from build123d import *

# Parameters (mm, degrees)
SKETCH1_W           = 139.7
SKETCH1_H           = 292.1
BOSS_EXTRUDE1_DEPTH = 6.35
FILLET1_R           = 12.7
SKETCH2_W           = 7.62
SKETCH2_H           = 29.0068
CUT_EXTRUDE1_DEPTH  = 6.35


with BuildPart() as part:
    # Sketch1 → Boss-Extrude1 (new body)
    with BuildSketch(Plane.XY):
        Rectangle(SKETCH1_W, SKETCH1_H)
    extrude(amount=BOSS_EXTRUDE1_DEPTH)

    # Fillet1
    fillet1_edges = [part.edges().sort_by_distance(p)[0] for p in [
        (69.85, -146.05, 3.175),
        (-69.85, -146.05, 3.175),
        (-69.85, 146.05, 3.175),
        (69.85, 146.05, 3.175),
    ]]
    fillet(fillet1_edges, radius=FILLET1_R)

    # Sketch2 → Cut-Extrude1 (cut)
    with BuildSketch(Plane.XY.offset(6.35)):
        with Locations((52.50815, 119.8626)):
            Rectangle(SKETCH2_W, SKETCH2_H)
        with BuildLine():
            Line((48.69815, 134.366), (56.31815, 134.366))
            ThreePointArc((56.31815, 134.366), (52.50815, 138.176), (48.69815, 134.366))
        make_face()
        with BuildLine():
            Line((48.69815, 105.3592), (56.31815, 105.3592))
            ThreePointArc((56.31815, 105.3592), (52.50815, 101.5492), (48.69815, 105.3592))
        make_face()
        with BuildLine():
            Line((48.69815, 65.6844), (48.69815, 94.6912))
            ThreePointArc((48.69815, 94.6912), (52.50815, 98.5012), (56.31815, 94.6912))
            Line((56.31815, 94.6912), (56.31815, 65.6844))
            ThreePointArc((56.31815, 65.6844), (52.50815, 61.8744), (48.69815, 65.6844))
        make_face()
        with BuildLine():
            Line((-56.31815, 65.6844), (-56.31815, 94.6912))
            ThreePointArc((-56.31815, 94.6912), (-52.50815, 98.5012), (-48.69815, 94.6912))
            Line((-48.69815, 94.6912), (-48.69815, 65.6844))
            ThreePointArc((-48.69815, 65.6844), (-52.50815, 61.8744), (-56.31815, 65.6844))
        make_face()
        with BuildLine():
            Line((-56.31815, 105.3592), (-56.31815, 134.366))
            ThreePointArc((-56.31815, 134.366), (-52.50815, 138.176), (-48.69815, 134.366))
            Line((-48.69815, 134.366), (-48.69815, 105.3592))
            ThreePointArc((-48.69815, 105.3592), (-52.50815, 101.5492), (-56.31815, 105.3592))
        make_face()
        with BuildLine():
            Line((48.69815, 26.0096), (48.69815, 55.0164))
            ThreePointArc((48.69815, 55.0164), (52.50815, 58.8264), (56.31815, 55.0164))
            Line((56.31815, 55.0164), (56.31815, 26.0096))
            ThreePointArc((56.31815, 26.0096), (52.50815, 22.1996), (48.69815, 26.0096))
        make_face()
        with BuildLine():
            Line((-56.31815, 26.0096), (-56.31815, 55.0164))
            ThreePointArc((-56.31815, 55.0164), (-52.50815, 58.8264), (-48.69815, 55.0164))
            Line((-48.69815, 55.0164), (-48.69815, 26.0096))
            ThreePointArc((-48.69815, 26.0096), (-52.50815, 22.1996), (-56.31815, 26.0096))
        make_face()
        with BuildLine():
            Line((48.69815, -13.6652), (48.69815, 15.3416))
            ThreePointArc((48.69815, 15.3416), (52.50815, 19.1516), (56.31815, 15.3416))
            Line((56.31815, 15.3416), (56.31815, -13.6652))
            ThreePointArc((56.31815, -13.6652), (52.50815, -17.4752), (48.69815, -13.6652))
        make_face()
        with BuildLine():
            Line((-56.31815, -13.6652), (-56.31815, 15.3416))
            ThreePointArc((-56.31815, 15.3416), (-52.50815, 19.1516), (-48.69815, 15.3416))
            Line((-48.69815, 15.3416), (-48.69815, -13.6652))
            ThreePointArc((-48.69815, -13.6652), (-52.50815, -17.4752), (-56.31815, -13.6652))
        make_face()
        with BuildLine():
            Line((-56.31815, -53.34), (-56.31815, -24.3332))
            ThreePointArc((-56.31815, -24.3332), (-52.50815, -20.5232), (-48.69815, -24.3332))
            Line((-48.69815, -24.3332), (-48.69815, -53.34))
            ThreePointArc((-48.69815, -53.34), (-52.50815, -57.15), (-56.31815, -53.34))
        make_face()
        with BuildLine():
            Line((48.69815, -53.34), (48.69815, -24.3332))
            ThreePointArc((48.69815, -24.3332), (52.50815, -20.5232), (56.31815, -24.3332))
            Line((56.31815, -24.3332), (56.31815, -53.34))
            ThreePointArc((56.31815, -53.34), (52.50815, -57.15), (48.69815, -53.34))
        make_face()
        with BuildLine():
            Line((48.69815, -93.0148), (48.69815, -64.008))
            ThreePointArc((48.69815, -64.008), (52.50815, -60.198), (56.31815, -64.008))
            Line((56.31815, -64.008), (56.31815, -93.0148))
            ThreePointArc((56.31815, -93.0148), (52.50815, -96.8248), (48.69815, -93.0148))
        make_face()
        with BuildLine():
            Line((-56.31815, -93.0148), (-56.31815, -64.008))
            ThreePointArc((-56.31815, -64.008), (-52.50815, -60.198), (-48.69815, -64.008))
            Line((-48.69815, -64.008), (-48.69815, -93.0148))
            ThreePointArc((-48.69815, -93.0148), (-52.50815, -96.8248), (-56.31815, -93.0148))
        make_face()
    extrude(amount=-CUT_EXTRUDE1_DEPTH, mode=Mode.SUBTRACT)


solid = part.part
Design review of the part built by this model. Coordinates are the model's own, in mm. A direction names the side the tool comes from. Give positions to 0.01 mm unless a question says otherwise; leave off trailing zeros. Loops run counter-clockwise (first coordinate to the right, second up) from the corner with the lowest first, then second, coordinate; pieces in that order, holes last. Notation, with made-up numbers: (52.5, 40) - (70.5, 40) arc R22 cw to (70.5, 77) - close; hole circle Ø10 at (29.5, 40.25). An arc over 180 degrees is marked (long way). Use CSV: the item, a comma, the result in double quotes. Start each with the question number.
1. Add section B-B (z = 4). Count the separate pieces of the cut face and the enclosed holes in it, plus the area to 3 significant figures.
2. Machinability: for faces 1 (the flat face through (48.698, 40, 3)), 2 (the flat face through (-1, -146.05, 3)), which of the approach directions +Z, -Z, +X, -X, +Y, -Y give a long, thin tool a straight path to every point of the face, cutting with its end or side? Answer none if there is none.
3. Add section A-A (y = -30.5). State the section outline as (x, z) points, plus the area to 3 significant figures.
4. Wall thickness on L1, parallel to X at y = 55, z = 0.75; L2, parallel to X at y = 58, z = 2.75; L3, parallel to Y at x = 64, z = 4: over which ranges is each line inside the solid? List them lowest first.
5. Draft analysis for pull direction X (two halves, no side actions). For faces 3 (the flat face through (-1, 2, 0)), 4 (the flat face through (69.85, -2, 3)), 5 (the flat face through (-48.698, -78, 3)), state which applies: released by +X, released by -X, zero draft, split by the parting line, or undercut.
6. Insertion check: P1, Ø1.5, axis at x = -39.5, y = 29.5, coming from the -Z side. The pin has a flat end and moves straight along its axis. Give the tip position at first contact, or say it passes through.
Results found:
1,separate pieces,"1"
1,enclosed holes,"12"
1,area,"37,500 mm²"
2,face 1,"+Z, -Z"
2,face 2,"+Z, -Z, +X, -X, -Y"
3,outline,"(-69.85, 0) - (-56.32, 0) - (-56.32, 6.35) - (-69.85, 6.35) - close; (-48.7, 0) - (48.7, 0) - (48.7, 6.35) - (-48.7, 6.35) - close; (56.32, 0) - (69.85, 0) - (69.85, 6.35) - (56.32, 6.35) - close"
3,area,"790 mm²"
4,L1,"x = -69.85 to -56.32, -48.7 to 48.7, 56.32 to 69.85"
4,L2,"x = -69.85 to -54.88, -50.14 to 50.14, 54.88 to 69.85"
4,L3,"y = -144.04 to 144.04"
5,face 3,"zero draft"
5,face 4,"released by +X"
5,face 5,"undercut"
6,P1,"stops at z = 0"
